The listing builds one solid part. Answer for the finished solid, in the listing's coordinates (mm). Give positions to 0.01 mm unless a question says otherwise; leave off trailing zeros. Order: outer loops, then holes, each group sorted by start corner. A loop starts at its lowest first (then second) coordinate and runs counter-clockwise, first axis right, second up. Notation, with made-up numbers: (7.25, 18) - (49.25, 18) arc R26 cw to (49.25, 43) - close; hole circle Ø5 at (25.25, -29.75). An arc over 180 degrees is marked (long way). Use CSV: the item, a comma, the result in double quotes.
```python
from build123d import *

# Parameters (mm, degrees)
BOSS_EXTRUDE1_DEPTH       = 6.35
F_6_CLEARANCE_HOLE1_D     = 3.6576
F_6_CLEARANCE_HOLE1_DEPTH = 25.4
F_6_CLEARANCE_HOLE1_TIP   = 1.0988539


with BuildPart() as part:
    # Sketch1 → Boss-Extrude1 (new body)
    with BuildSketch(Plane(origin=(0, 0, 0), x_dir=(1, 0, 0), z_dir=(0, 1, 0))):
        with BuildLine():
            Line((166.494481955, 130.873744419), (240.574340444, 200.406))
            ThreePointArc((240.574340444, 200.406), (0, 304.546), (-240.574340444, 200.406))
            Line((-240.574340444, 200.406), (-166.494481955, 130.873744419))
            ThreePointArc((-166.494481955, 130.873744419), (0, 202.946), (166.494481955, 130.873744419))
        make_face()
    extrude(amount=BOSS_EXTRUDE1_DEPTH)

    # #6 Clearance Hole1
    with Locations(Plane(origin=(-50.8, 6.35, -253.746255929), x_dir=(0, 0, 1), z_dir=(0, 1, 0))):
        with Locations((0, 0), (0, 101.6)):
            Hole(F_6_CLEARANCE_HOLE1_D / 2, depth=F_6_CLEARANCE_HOLE1_DEPTH)
            with Locations((0, 0, -(F_6_CLEARANCE_HOLE1_DEPTH + F_6_CLEARANCE_HOLE1_TIP / 2))):  # 118° drill point
                Cone(0, F_6_CLEARANCE_HOLE1_D / 2, F_6_CLEARANCE_HOLE1_TIP, mode=Mode.SUBTRACT)


solid = part.part
```
Item 1: The part is cut by section C-C (x = 3). Give the vertices of the cut face in (y, z), and give its area (3 significant figures).
Taken from the geometry:
outline,"(0, -304.53) - (6.35, -304.53) - (6.35, -202.93) - (0, -202.93) - close"
area,"645 mm^2"
Item 2: The part is cut by section B-B (y = 5.25). Give the vertices of the cut face in (x, z), and give its area (3 significant figures).
Taken from the geometry:
outline,"(-240.57, -200.41) arc R329.95 ccw to (240.57, -200.41) - (166.49, -130.87) arc R228.35 cw to (-166.49, -130.87) - close; hole circle Ø3.66 at (-50.8, -253.75); hole circle Ø3.66 at (50.8, -253.75)"
area,"46,300 mm^2"
Item 3: The part is cut by section D-D (z = -289.5). Give the vertices of the cut face in (x, y).
Taken from the geometry:
outline,"(-98.5, 0) - (98.5, 0) - (98.5, 6.35) - (-98.5, 6.35) - close"
Item 4: Find the intervals of material crossed by line 1 along X through (y, z) = (2.25, -253); line 2 along X through (y, z) = (1, -180.5); line 3 along X through (y, z) = (3.5, -183), in increasing order.
Taken from the geometry:
line 1,"-177.08 to -52.47, -49.13 to 49.13, 52.47 to 177.08"
line 2,"-219.37 to -98.73, 98.73 to 219.37"
line 3,"-222.03 to -93.33, 93.33 to 222.03"
Item 5: The part is cut by section A-A (z = -185). Give the vertices of the cut face in (x, y).
Taken from the geometry:
outline,"(-224.16, 0) - (-88.73, 0) - (-88.73, 6.35) - (-224.16, 6.35) - close; (88.73, 0) - (224.16, 0) - (224.16, 6.35) - (88.73, 6.35) - close"
